```python
from build123d import *

# Parameters (mm, degrees)
SKETCH1_W           = 605
SKETCH1_H           = 425
BOSS_EXTRUDE1_DEPTH = 20
BOSS_EXTRUDE2_DEPTH = 246
SKETCH3_W           = 30
SKETCH3_H           = 53
CUT_EXTRUDE1_DEPTH  = 423
SKETCH4_R           = 4
CUT_EXTRUDE2_DEPTH  = 549.5
SKETCH5_W           = 230
SKETCH5_H           = 53
CUT_EXTRUDE3_DEPTH  = 220
SKETCH6_W           = 458
SKETCH6_H           = 30
BOSS_EXTRUDE3_DEPTH = 15
SKETCH7_W           = 458
SKETCH7_H           = 28
BOSS_EXTRUDE4_DEPTH = 4.3


with BuildPart() as part:
    # Sketch1 → Boss-Extrude1 (new body)
    with BuildSketch(Plane(origin=(0, 0, 0), x_dir=(1, 0, 0), z_dir=(0, 1, 0))):
        Rectangle(SKETCH1_W, SKETCH1_H)
    extrude(amount=-BOSS_EXTRUDE1_DEPTH)

    # Sketch2 → Boss-Extrude2 (add, symmetric)
    with BuildSketch(Plane(origin=(0, 0, 0), x_dir=(0, 0, -1), z_dir=(1, 0, 0))):
        with BuildLine():
            Line((203.7, 0), (-209.5, 0))
            Line((-209.5, 0), (-209.5, 53))
            Line((-209.5, 53), (173.7, 53))
            ThreePointArc((173.7, 53), (194.913203436, 44.213203436), (203.7, 23))
            Line((203.7, 23), (203.7, 0))
        make_face()
    extrude(amount=BOSS_EXTRUDE2_DEPTH, both=True)

    # Sketch3 → Cut-Extrude1 (cut, through all)
    with BuildSketch(Plane.XY.offset(209.5)):
        with Locations((-216, 26.5)):
            Rectangle(SKETCH3_W, SKETCH3_H)
        with Locations((-168, 26.5)):
            Rectangle(SKETCH3_W, SKETCH3_H)
        with Locations((-120, 26.5)):
            Rectangle(SKETCH3_W, SKETCH3_H)
        with Locations((-72, 26.5)):
            Rectangle(SKETCH3_W, SKETCH3_H)
        with Locations((-24, 26.5)):
            Rectangle(SKETCH3_W, SKETCH3_H)
        with Locations((24, 26.5)):
            Rectangle(SKETCH3_W, SKETCH3_H)
        with Locations((72, 26.5)):
            Rectangle(SKETCH3_W, SKETCH3_H)
        with Locations((120, 26.5)):
            Rectangle(SKETCH3_W, SKETCH3_H)
        with Locations((168, 26.5)):
            Rectangle(SKETCH3_W, SKETCH3_H)
        with Locations((216, 26.5)):
            Rectangle(SKETCH3_W, SKETCH3_H)
    extrude(amount=-CUT_EXTRUDE1_DEPTH, mode=Mode.SUBTRACT)

    # Sketch4 → Cut-Extrude2 (cut, through all)
    with BuildSketch(Plane.ZY.offset(246)):
        with Locations((-44.5, 41)):
            Circle(SKETCH4_R)
    extrude(amount=-CUT_EXTRUDE2_DEPTH, mode=Mode.SUBTRACT)

    # Sketch5 → Cut-Extrude3 (cut, symmetric)
    with BuildSketch(Plane(origin=(0, 0, 0), x_dir=(0, 0, -1), z_dir=(1, 0, 0))):
        with Locations((-94.5, 26.5)):
            Rectangle(SKETCH5_W, SKETCH5_H)
    extrude(amount=CUT_EXTRUDE3_DEPTH, both=True, mode=Mode.SUBTRACT)

    # Sketch6 → Boss-Extrude3 (add)
    with BuildSketch(Plane(origin=(0, 0, 0), x_dir=(1, 0, 0), z_dir=(0, 1, 0))):
        with Locations((0, -189.5)):
            Rectangle(SKETCH6_W, SKETCH6_H)
    extrude(amount=BOSS_EXTRUDE3_DEPTH)

    # Sketch7 → Boss-Extrude4 (add)
    with BuildSketch(Plane(origin=(0, 0, 0), x_dir=(1, 0, 0), z_dir=(0, 1, 0))):
        with Locations((0, -96.5)):
            Rectangle(SKETCH7_W, SKETCH7_H)
    extrude(amount=BOSS_EXTRUDE4_DEPTH)


solid = part.part
```
Check sheet for the modelled part. Datum: model origin and axes. Units: mm. A direction names the side the tool comes from. Round coordinates to 2 decimals unless told otherwise and drop trailing zeros. Loops run counter-clockwise (first coordinate to the right, second up) from the corner with the lowest first, then second, coordinate; pieces in that order, holes last. Notation, with made-up numbers: (-28.5, 75.5) - (18.5, 75.5) arc R23 ccw to (18.5, 113.5) - close; hole circle Ø3 at (20.5, -29). An arc over 180 degrees is marked (long way). Write item = value, one per line. Start each with the question number.
Q1. Section check B-B (x = 26). Record the boundary of the cut face in (y, z), plus the area to 3 significant figures.
Q2. Thickness scan on L1, parallel to X at y = 20.5, z = 160.5; L2, parallel to Y at x = -142.5, z = -44.5; L3, parallel to Z at x = -198, y = 23. Record the ranges inside material, lowest first.
Q3. Section check A-A (z = 65). Record the boundary of the cut face in (x, y), plus the area to 3 significant figures.
Q4. Depth check by flat-ended pin: P1, Ø10.5, axis at y = 41, z = -44.5, coming from the -X side; P2, Ø7.5, axis at x = -241.5, y = 16.5, coming from the +Z side; P3, Ø4.5, axis at y = 9.5, z = 196.5, coming from the +X side. Enter the tip coordinate at first touch or a pass-through.
Q5. Access from +Z, -Z, +X, -X, +Y, -Y to the whole of each face (thin tool, end or side, straight path). Record for faces 1 (the face through (239, 26, 209.5)), 2 (the face through (9, 26, -111)), 3 (the face through (-48, 12, -203.7)), 4 (the face through (-246, 27, 0)).
Q6. Release check for a two-part mould opening along Z. For faces 5 (the face through (0, 12, -203.7)), 6 (the face through (105, 26, -111)), 7 (the face through (-238, 26, 209.5)), 8 (the face through (-96, 26, -20.5)) record: pulls with the +Z half, pulls with the -Z half, needs draft (parallel to the pull), parting line crosses it, or undercut.
Q7. Section check C-C (y = 29.5). Count the separate pieces of the cut face and the enclosed holes in it, plus the area to 3 significant figures.
Derived:
q1.outline = (-20, -212.5) - (0, -212.5) - (0, 82.5) - (4.3, 82.5) - (4.3, 110.5) - (0, 110.5) - (0, 174.5) - (15, 174.5) - (15, 204.5) - (0, 204.5) - (0, 212.5) - (-20, 212.5) - close
q1.area = 9,070 mm^2
q2.L1 = -246 to -231, 231 to 246
q2.L2 = -20 to 37, 45 to 53
q2.L3 = -203.7 to -20.5
q3.outline = (-302.5, -20) - (302.5, -20) - (302.5, 0) - (246, 0) - (246, 53) - (231, 53) - (231, 0) - (-231, 0) - (-231, 53) - (-246, 53) - (-246, 0) - (-302.5, 0) - close
q3.area = 13,700 mm^2
q4.P1 = -246
q4.P2 = 209.5
q4.P3 = 246
q5.face_1 = +Z, +X, -X, +Y
q5.face_2 = -Z, +Y
q5.face_3 = -Z, +X, -X, +Y
q5.face_4 = +Z, -Z, -X, +Y
q6.face_5 = pulls with the -Z half
q6.face_6 = needs draft
q6.face_7 = pulls with the +Z half
q6.face_8 = undercut
q7.separate_pieces = 11
q7.enclosed_holes = 0
q7.area = 41,900 mm^2
